from build123d import *

# Parameters (mm, degrees)
SKETCH1_W               = 50
SKETCH1_H               = 34
BOSS_EXTRUDE1_DEPTH     = 60
CUT_EXTRUDE1_DEPTH      = 68.186308129
SKETCH3_R               = 2.25
CUT_EXTRUDE2_DEPTH      = 74.35529974
CUT_EXTRUDE3_DEPTH      = 24.8
CHAMFER1_SIZE           = 1
CHAMFER1_SIZE_2         = 1.220120443
SKETCH5_W               = 200
SKETCH5_H               = 34
BOSS_EXTRUDE2_DEPTH     = 6
BOSS_EXTRUDE3_DEPTH     = 1
FILLET1_R               = 5
FILLET2_R               = 5
SKETCH7_R               = 2.25
CUT_EXTRUDE4_DEPTH      = 4
SKETCH8_R               = 2.25
CUT_EXTRUDE5_DEPTH      = 119.882294729
LPATTERN1_COUNT         = 2
LPATTERN1_PITCH         = 25
MIRROR4_COPY_1_SKETCH_R = 2.25
MIRROR4_COPY_1_DEPTH    = 4
MIRROR4_COPY_2_SKETCH_R = 2.25
MIRROR4_COPY_2_DEPTH    = 119.882294729
CUT_EXTRUDE6_DEPTH      = 4
SKETCH10_R              = 7
BOSS_EXTRUDE4_DEPTH     = 14
SKETCH11_R              = 7
SKETCH11_R_2            = 4.15
BOSS_EXTRUDE5_DEPTH     = 20
CHAMFER2_SIZE           = 10
CHAMFER2_SIZE2          = 0.174550649
CHAMFER3_SIZE           = 10


with BuildPart() as part:
    # Sketch1 → Boss-Extrude1 (new body)
    with BuildSketch(Plane(origin=(0, 0, 0), x_dir=(1, 0, 0), z_dir=(0, 1, 0))):
        Rectangle(SKETCH1_W, SKETCH1_H)
    extrude(amount=BOSS_EXTRUDE1_DEPTH)

    # Sketch2 → Cut-Extrude1 (cut, through all)
    with BuildSketch(Plane(origin=(0, 60, 0), x_dir=(1, 0, 0), z_dir=(0, 1, 0))):
        with BuildLine():
            Line((-3.75, 3.5), (-7, -2.8))
            Line((-7, -2.8), (-7, -9.8))
            Line((-7, -9.8), (-15.5, -9.8))
            Line((-15.5, -9.8), (-15.5, -14))
            Line((-15.5, -14), (15.5, -14))
            Line((15.5, -14), (15.5, -9.8))
            Line((15.5, -9.8), (7, -9.8))
            Line((7, -9.8), (7, -2.8))
            Line((7, -2.8), (3.75, 3.5))
            ThreePointArc((3.75, 3.5), (0, 14.75), (-3.75, 3.5))
        make_face()
    extrude(amount=-CUT_EXTRUDE1_DEPTH, mode=Mode.SUBTRACT)

    # Sketch3 → Cut-Extrude2 (cut, through all)
    with BuildSketch(Plane.XY.offset(17)):
        with Locations((-11, 50)):
            Circle(SKETCH3_R)
        with Locations((11, 50)):
            Circle(SKETCH3_R)
    extrude(amount=-CUT_EXTRUDE2_DEPTH, mode=Mode.SUBTRACT)

    # Sketch4 → Cut-Extrude3 (cut)
    with BuildSketch(Plane(origin=(0, 0, -17), x_dir=(-1, 0, 0), z_dir=(0, 0, -1))):
        Polygon((14.75, 52.165063509), (11, 54.330127019), (7.25, 52.165063509), (7.25, 47.834936491), (11, 45.669872981), (14.75, 47.834936491), align=None)
        Polygon((-7.25, 47.834936491), (-7.25, 52.165063509), (-11, 54.330127019), (-14.75, 52.165063509), (-14.75, 47.834936491), (-11, 45.669872981), align=None)
    extrude(amount=-CUT_EXTRUDE3_DEPTH, mode=Mode.SUBTRACT)

    # Chamfer1
    # the kernel refuses this chamfer: 1.220120443, 1 mm, written as the material it takes off along each edge
    with BuildSketch(Plane(origin=(-7, 62.571682988, 9.8), x_dir=(-1, 0, 0), z_dir=(0, -1, 0)), Plane(origin=(7, 62.571682988, 9.8), x_dir=(0, 0, -1), z_dir=(0, -1, 0))) as chamfer1_piece_1:
        Polygon((CHAMFER1_SIZE, 0), (0, CHAMFER1_SIZE), (0, 0), align=None)
    extrude(amount=65.143365976, mode=Mode.SUBTRACT)
    with BuildSketch(Plane(origin=(-3.75, 63.150527813, -3.5), x_dir=(-0.45846324589157744, 0, 0.8887133689590581), z_dir=(0, -1, 0))) as chamfer1_piece_2:
        with BuildLine():
            Line((CHAMFER1_SIZE_2, 0), (-0.278286757, 1.065574765))
            ThreePointArc((-0.278286757, 1.065574765), (-0.120412167, 0.557139368), (0, 0))
            Line((0, 0), (CHAMFER1_SIZE_2, 0))
        make_face()
    extrude(amount=66.301055626, mode=Mode.SUBTRACT)
    with BuildSketch(Plane(origin=(3.75, 63.795705698, -3.5), x_dir=(0.7235959376340886, 0, -0.6902238180760238), z_dir=(0, -1, 0))) as chamfer1_piece_3:
        with BuildLine():
            Line((1.475268649, 0), (-CHAMFER1_SIZE * 0.281668992416, CHAMFER1_SIZE * 0.959511635527))
            Line((-CHAMFER1_SIZE * 0.281668992416, CHAMFER1_SIZE * 0.959511635527), (0, 0))
            ThreePointArc((0, 0), (0.759242358, 0.043643641), (1.475268649, 0))
        make_face()
    extrude(amount=67.591411396, mode=Mode.SUBTRACT)

    # Sketch5 → Boss-Extrude2 (add)
    with BuildSketch(Plane.XZ):
        Rectangle(SKETCH5_W, SKETCH5_H)
    extrude(amount=BOSS_EXTRUDE2_DEPTH)

    # Sketch6 → Boss-Extrude3 (add, symmetric)
    with BuildSketch(Plane.XY):
        Polygon((-100, 0), (-25, 25), (-25, 0), align=None)
    boss_extrude3 = extrude(amount=BOSS_EXTRUDE3_DEPTH, both=True)

    # Mirror3: Boss-Extrude3 across plane
    add(boss_extrude3.mirror(Plane(origin=(0, 0, 0), x_dir=(0, 0, 1), z_dir=(1, 0, 0))))

    # Fillet1
    # the kernel refuses this fillet: 5 mm, written as the material it adds along each edge
    with BuildSketch(Plane(origin=(-12.5, 0, -1), x_dir=(0, 0, -1), z_dir=(-1, 0, 0))) as fillet1_piece_1_section:
        with BuildLine():
            CenterArc((FILLET1_R, -FILLET1_R), FILLET1_R, 90, 90)
            Line((0, -FILLET1_R), (0, 0))
            Line((0, 0), (FILLET1_R, 0))
        make_face()
    fillet1_piece_1 = extrude(amount=87.5, mode=Mode.PRIVATE)
    fillet1_piece_1 = split(fillet1_piece_1, bisect_by=Plane(origin=(-21.25, 26.25, -1), z_dir=(0.31622776601683794, -0.9486832980505139, 0)), keep=Keep.TOP, mode=Mode.PRIVATE)
    add(fillet1_piece_1)
    with BuildSketch(Plane(origin=(-12.5, 0, 1), x_dir=(0, 0, 1), z_dir=(-1, 0, 0))) as fillet1_piece_2_section:
        with BuildLine():
            CenterArc((FILLET1_R, FILLET1_R), FILLET1_R, 180, 90)
            Line((0, FILLET1_R), (0, 0))
            Line((0, 0), (FILLET1_R, 0))
        make_face()
    fillet1_piece_2 = extrude(amount=87.5, mode=Mode.PRIVATE)
    fillet1_piece_2 = split(fillet1_piece_2, bisect_by=Plane(origin=(-21.25, 26.25, 1), z_dir=(0.31622776601683794, -0.9486832980505139, 0)), keep=Keep.TOP, mode=Mode.PRIVATE)
    add(fillet1_piece_2)
    with BuildSketch(Plane(origin=(12.5, 0, 1), x_dir=(0, 0, 1), z_dir=(1, 0, 0))) as fillet1_piece_3_section:
        with BuildLine():
            CenterArc((FILLET1_R, -FILLET1_R), FILLET1_R, 90, 90)
            Line((0, -FILLET1_R), (0, 0))
            Line((0, 0), (FILLET1_R, 0))
        make_face()
    fillet1_piece_3 = extrude(amount=87.5, mode=Mode.PRIVATE)
    fillet1_piece_3 = split(fillet1_piece_3, bisect_by=Plane(origin=(21.25, 26.25, 1), z_dir=(-0.31622776601683794, -0.9486832980505139, 0)), keep=Keep.TOP, mode=Mode.PRIVATE)
    add(fillet1_piece_3)
    with BuildSketch(Plane(origin=(12.5, 0, -1), x_dir=(0, 0, -1), z_dir=(1, 0, 0))) as fillet1_piece_4_section:
        with BuildLine():
            CenterArc((FILLET1_R, FILLET1_R), FILLET1_R, 180, 90)
            Line((0, FILLET1_R), (0, 0))
            Line((0, 0), (FILLET1_R, 0))
        make_face()
    fillet1_piece_4 = extrude(amount=87.5, mode=Mode.PRIVATE)
    fillet1_piece_4 = split(fillet1_piece_4, bisect_by=Plane(origin=(21.25, 26.25, -1), z_dir=(-0.31622776601683794, -0.9486832980505139, 0)), keep=Keep.TOP, mode=Mode.PRIVATE)
    add(fillet1_piece_4)

    # Fillet2
    fillet2_edges = [part.edges().sort_by_distance(p)[0] for p in [
        (-25, 25, 0),
        (25, 25, 0),
        (25, 15, -1),
        (25, 0, -11.5),
        (25, 15, 1),
        (25, 1.464466094, 2.464466094),
        (25, 1.464466094, -2.464466094),
        (-25, 15, -1),
        (-25, 15, 1),
        (-25, 0, 11.5),
        (-25, 1.464466094, 2.464466094),
        (-25, 1.464466094, -2.464466094),
        (25, 0, 11.5),
        (-25, 0, -11.5),
    ]]
    fillet(fillet2_edges, radius=FILLET2_R)

    # Sketch7 → Cut-Extrude4 (cut)
    with BuildSketch(Plane.XZ.offset(6)):
        with Locations(Location((-75, 10, 0), (0, 0, 270))):
            Circle(SKETCH7_R)
        with Locations(Location((-75, -10, 0), (0, 0, 270))):
            Circle(SKETCH7_R)
    cut_extrude4 = extrude(amount=-CUT_EXTRUDE4_DEPTH, mode=Mode.SUBTRACT)

    # Sketch8 → Cut-Extrude5 (cut, through all)
    with BuildSketch(Plane(origin=(0, -2, 0), x_dir=(-1, 0, 0), z_dir=(0, -1, 0))):
        with Locations(Location((75, -10, 0), (0, 0, 90))):
            Circle(SKETCH8_R)
        with Locations(Location((75, 10, 0), (0, 0, 90))):
            Circle(SKETCH8_R)
    cut_extrude5 = extrude(amount=-CUT_EXTRUDE5_DEPTH, mode=Mode.SUBTRACT)

    # LPattern1: Cut-Extrude4, Cut-Extrude5 ×2
    with Locations(*[(i * LPATTERN1_PITCH, 0, 0) for i in range(1, LPATTERN1_COUNT)]):
        add(cut_extrude4, mode=Mode.SUBTRACT)
        add(cut_extrude5, mode=Mode.SUBTRACT)

    # Mirror4: Cut-Extrude4, Cut-Extrude5 across plane
    add(cut_extrude4.mirror(Plane(origin=(0, 0, 0), x_dir=(0, 0, 1), z_dir=(1, 0, 0))), mode=Mode.SUBTRACT)
    add(cut_extrude5.mirror(Plane(origin=(0, 0, 0), x_dir=(0, 0, 1), z_dir=(1, 0, 0))), mode=Mode.SUBTRACT)

    # Mirror4 copy 1 sketch → Mirror4 copy 1 (cut)
    with BuildSketch(Plane(origin=(-25, -6, 0), x_dir=(-1, 0, 0), z_dir=(0, -1, 0))):
        with Locations((-75, -10)):
            Circle(MIRROR4_COPY_1_SKETCH_R)
        with Locations((-75, 10)):
            Circle(MIRROR4_COPY_1_SKETCH_R)
    extrude(amount=-MIRROR4_COPY_1_DEPTH, mode=Mode.SUBTRACT)

    # Mirror4 copy 2 sketch → Mirror4 copy 2 (cut, through all)
    with BuildSketch(Plane(origin=(-25, -2, 0), x_dir=(1, 0, 0), z_dir=(0, -1, 0))):
        with Locations((75, 10)):
            Circle(MIRROR4_COPY_2_SKETCH_R)
        with Locations((75, -10)):
            Circle(MIRROR4_COPY_2_SKETCH_R)
    extrude(amount=-MIRROR4_COPY_2_DEPTH, mode=Mode.SUBTRACT)

    # Sketch9 → Cut-Extrude6 (cut)
    with BuildSketch(Plane(origin=(0, 0, 0), x_dir=(1, 0, 0), z_dir=(0, 1, 0))):
        with BuildLine():
            Line((4.208463246, 2.611286631), (4.817498401, 4.518265559))
            ThreePointArc((4.817498401, 4.518265559), (-0.187957188, 14.747173128), (-4.56940629, 4.235844027))
            Line((-4.56940629, 4.235844027), (-4.309380379, 2.415662651))
            Line((-4.309380379, 2.415662651), (-7, -2.8))
            Line((-7, -2.8), (-7, -8.8))
            Line((-7, -8.8), (-8, -9.8))
            Line((-8, -9.8), (-15.5, -9.8))
            Line((-15.5, -9.8), (-15.5, -14))
            Line((-15.5, -14), (15.5, -14))
            Line((15.5, -14), (15.5, -9.8))
            Line((15.5, -9.8), (8, -9.8))
            Line((8, -9.8), (7, -8.8))
            Line((7, -8.8), (7, -2.8))
            Line((7, -2.8), (4.208463246, 2.611286631))
        make_face()
    extrude(amount=-CUT_EXTRUDE6_DEPTH, mode=Mode.SUBTRACT)

    # Sketch10 → Boss-Extrude4 (add)
    with BuildSketch(Plane(origin=(0, 0, -17), x_dir=(-1, 0, 0), z_dir=(0, 0, -1))):
        with Locations(Location((0, 19, 0), (0, 0, 180))):
            Circle(SKETCH10_R)
    extrude(amount=BOSS_EXTRUDE4_DEPTH)

    # Sketch11 → Boss-Extrude5 (add)
    with BuildSketch(Plane(origin=(0, 0, -31), x_dir=(-1, 0, 0), z_dir=(0, 0, -1))):
        with Locations(Location((0, 19, 0), (0, 0, 180))):
            Circle(SKETCH11_R)
        with Locations((0, 19)):
            Circle(SKETCH11_R_2, mode=Mode.SUBTRACT)
    extrude(amount=BOSS_EXTRUDE5_DEPTH)

    # Chamfer2
    chamfer2_edges = [part.edges().sort_by_distance(p)[0] for p in [
        (4.15, 19, -31),
    ]]
    chamfer2_side = [part.faces().sort_by_distance(p)[0] for p in [
        (4.15, 19, -41),
    ]]
    chamfer(chamfer2_edges, length=CHAMFER2_SIZE, length2=CHAMFER2_SIZE2, reference=chamfer2_side[0])

    # Chamfer3
    chamfer3_edges = [part.edges().sort_by_distance(p)[0] for p in [
        (-7, 19, -17),
    ]]
    chamfer(chamfer3_edges, length=CHAMFER3_SIZE)


solid = part.part
Work out the finished part from the listing and answer in its coordinate system (mm). A direction names the side the tool comes from. Coordinates: 2 decimals unless noted, no trailing zeros. Loops run counter-clockwise (first coordinate to the right, second up) from the corner with the lowest first, then second, coordinate; pieces in that order, holes last. Notation, with made-up numbers: (-29.75, 42) -> (29.25, 42) arc R23 ccw to (29.25, 77) -> close; hole circle Ø5 at (-15.5, -37). An arc over 180 degrees is marked (long way). Write each question's results on one line, items separated by ' | '. Start each with the question number.
1) For faces 1 (the flat face through (-65, 0, -11)), 2 (the conical face through (-1.874, 15.397, -35.93)), 3 (the cylindrical face through (27, 14, -2)), determine the directions among +Z, -Z, +X, -X, +Y, -Y from which every point of the face is accessible in a straight line to the end or side of a thin tool.
2) Find section B-B on x = 50. Determine the outline of the cut face in (y, z), then the cut area to 3 significant figures.
3) Consider line 1 along X through (y, z) = (52, -15); line 2 along Z through (x, y) = (50, -1); line 3 along X through (y, z) = (43, -8). Determine where each line is inside the solid, lowest interval first.
4) Find section C-C on x = 75. Determine the outline of the cut face in (y, z).
5) Flat-ended cylindrical pins translate along their axes: P1, Ø6.5, axis at x = 1.5, y = 18, coming from the -Z side; P2, Ø5.5, axis at x = -55, z = -13.5, coming from the +Y side; P3, Ø3.5, axis at x = -75, z = 10, coming from the -Y side; P4, Ø5.5, axis at x = 45, y = 13.5, coming from the -Z side. Find the tip coordinate at first contact, or state that the pin passes through.
6) The mould has two halves that part along X. Classify faces 4 (the cylindrical face through (27, 1, -12)), 5 (the flat face through (-1, -6, 0)), 6 (the cylindrical face through (-77.196, -3.042, 10.488)): pulls with the +X half, pulls with the -X half, needs draft (parallel to the pull), parting line crosses it, or undercut.
7) Find section A-A on y = 56.5. Determine the outline of the cut face in (x, z).
Response values:
1) face 1: -Z, -X, +Y | face 2: -Z | face 3: -Z, +X, +Y
2) outline: (-6, -17) -> (0, -17) -> (0, -12.25) -> (-6, -12.25) -> close; (-6, -7.75) -> (0, -7.75) -> (0, -6) arc R5 cw to (5, -1) -> (16.67, -1) -> (16.67, 1) -> (5, 1) arc R5 cw to (0, 6) -> (0, 7.75) -> (-6, 7.75) -> close; (-6, 12.25) -> (0, 12.25) -> (0, 17) -> (-6, 17) -> close | area: 194 mm^2
3) line 1: x = -25 to -14.75, -7.25 to 7.25, 14.75 to 25 | line 2: z = -17 to -12.25, -7.75 to 7.75, 12.25 to 17 | line 3: x = -25 to -6.23, 6.23 to 25
4) outline: (-6, -17) -> (0, -17) -> (0, -12.25) -> (-6, -12.25) -> close; (-6, -7.75) -> (0, -7.75) -> (0, -6) arc R5 cw to (5, -1) -> (8.33, -1) -> (8.33, 1) -> (5, 1) arc R5 cw to (0, 6) -> (0, 7.75) -> (-6, 7.75) -> close; (-6, 12.25) -> (0, 12.25) -> (0, 17) -> (-6, 17) -> close
5) P1: stops at z = -51 | P2: stops at y = 0 | P3: passes through | P4: stops at z = -1
6) face 4: pulls with the +X half | face 5: needs draft | face 6: undercut
7) outline: (-25, -17) -> (25, -17) -> (25, 17) -> (-25, 17) -> close; hole (-15.5, 9.8) -> (-8, 9.8) -> (-7, 8.8) -> (-7, 2.8) -> (-4.31, -2.42) -> (-4.57, -4.24) arc R6.25 ccw (long way) to (4.82, -4.52) -> (4.21, -2.61) -> (7, 2.8) -> (7, 8.8) -> (8, 9.8) -> (15.5, 9.8) -> (15.5, 14) -> (-15.5, 14) -> close
